Here's how the part is built. I have some questions about the finished solid (model axes, mm). Face numbers are marked on the shaded views. A direction names the side the tool comes from. Coordinates: 2 decimals unless noted, no trailing zeros. Write each loop counter-clockwise with the first axis right and the second up, starting at its lowest first coordinate (ties: lowest second). Pieces come first, ordered by that corner, then holes.
(1) Imagine slicing it at C-C, the plane x = -12.5. List the corners of the cut face in (y, z) for me, plus the area to 3 significant figures.
(2) Imagine slicing it at D-D, the plane z = -7.25. List the corners of the cut face in (x, y) for me.
(3) Imagine slicing it at B-B, the plane x = -7.5. List the corners of the cut face in (y, z) for me, plus the area to 3 significant figures.
(4) Imagine slicing it at A-A, the plane y = 51. List the corners of the cut face in (x, z) for me.
(5) Which directions (+Z, -Z, +X, -X, +Y, -Y) give clear straight access to the entire face, cutting with the end or side of a thin tool? Please do the marked faces 4, 5 and 6.
(6) For pin 1 Ø1 at (y, z) = (38.5, 6) entering from -X; pin 2 Ø1.6 at (x, z) = (24.5, -0.5) entering from +Y; pin 3 Ø4.5 at (y, z) = (30.5, 8.5) entering from +X, each with a flat end and sliding along its axis, tell me the tip position at first contact or that it passes through.
(7) Please list where these lines run through material, in increasing order: probe 1 along Y at (x, z) = (-13.25, -5); probe 2 along X at (y, z) = (2.75, 0); probe 3 along Z at (x, y) = (-10.75, 4).
(8) Thinking about a two-plate mould opening in Y: for the marked faces 1, 2 and 3, which applies, released by +Y, released by -Y, zero draft, split by the parting line, or undercut?
```python
from build123d import *

# Parameters (mm, degrees)
ESQUISSE1_W                                 = 45
ESQUISSE1_H                                 = 30
BOSS_EXTRU_1_DEPTH                          = 8
ESQUISSE5_W                                 = 30
ESQUISSE5_H                                 = 48
BOSS_EXTRU_3_DEPTH                          = 32
ENL_V_MAT_EXTRU_1_DEPTH                     = 27
ESQUISSE14_W                                = 6
ESQUISSE14_H                                = 8
ENL_V_MAT_EXTRU_2_DEPTH                     = 65.600696591
D_GAGEMENT_M31_D                            = 3.2
D_GAGEMENT_M31_DEPTH                        = 7
D_GAGEMENT_M31_TIP                          = 0.96137699
ESQUISSE16_W                                = 30
ESQUISSE16_H                                = 48
ESQUISSE16_R                                = 3.5
BOSS_EXTRU_4_DEPTH                          = 5
CONG_1_R                                    = 2
ESQUISSE17_W                                = 10
ESQUISSE17_H                                = 10
ENL_V_MAT_EXTRU_3_DEPTH                     = 2
BOSS_EXTRU_5_START                          = 2
ESQUISSE18_R                                = 6
ESQUISSE18_R_2                              = 3.5
BOSS_EXTRU_5_DEPTH                          = 2
FRAISAGE_POUR_VIS_T_TE_FRAIS_E_M31_AT_COUNT = 2
FRAISAGE_POUR_VIS_T_TE_FRAIS_E_M31_AT_PITCH = 15
ESQUISSE24_W                                = 8
ESQUISSE24_H                                = 8
BOSS_EXTRU_6_DEPTH                          = 2.6


with BuildPart() as part:
    # Esquisse1 → Boss.-Extru.1 (new body)
    with BuildSketch(Plane(origin=(0, 0, 0), x_dir=(1, 0, 0), z_dir=(0, 1, 0))):
        with Locations((6, 0)):
            Rectangle(ESQUISSE1_W, ESQUISSE1_H)
    extrude(amount=BOSS_EXTRU_1_DEPTH)

    # Esquisse5 → Boss.-Extru.3 (add)
    with BuildSketch(Plane.ZY.offset(16.5)):
        with Locations((0, 32)):
            Rectangle(ESQUISSE5_W, ESQUISSE5_H)
    extrude(amount=-BOSS_EXTRU_3_DEPTH)

    # Esquisse6 → Enl_v. mat.-Extru.1 (cut)
    with BuildSketch(Plane.ZY.offset(16.5)):
        Polygon((10.25, 48), (4, 48), (4, 56), (-4, 56), (-4, 48), (-10.25, 48), (-10.25, 8), (10.25, 8), align=None)
    extrude(amount=-ENL_V_MAT_EXTRU_1_DEPTH, mode=Mode.SUBTRACT)

    # Esquisse14 → Enl_v. mat.-Extru.2 (cut, through all)
    with BuildSketch(Plane(origin=(0, 56, 0), x_dir=(1, 0, 0), z_dir=(0, 1, 0))):
        with Locations((16.5, 0)):
            Rectangle(ESQUISSE14_W, ESQUISSE14_H)
    extrude(amount=-ENL_V_MAT_EXTRU_2_DEPTH, mode=Mode.SUBTRACT)

    # D_gagement M31
    with Locations(Plane.ZY.offset(16.5)):
        with Locations((5, 4), (-5, 4)):
            Hole(D_GAGEMENT_M31_D / 2, depth=D_GAGEMENT_M31_DEPTH)
            with Locations((0, 0, -(D_GAGEMENT_M31_DEPTH + D_GAGEMENT_M31_TIP / 2))):  # 118° drill point
                Cone(0, D_GAGEMENT_M31_D / 2, D_GAGEMENT_M31_TIP, mode=Mode.SUBTRACT)

    # Esquisse16 → Boss.-Extru.4 (add)
    with BuildSketch(Plane(origin=(28.5, 0, 0), x_dir=(0, 0, -1), z_dir=(1, 0, 0))):
        with Locations((0, 32)):
            Rectangle(ESQUISSE16_W, ESQUISSE16_H)
        with Locations((0, 38)):
            Circle(ESQUISSE16_R, mode=Mode.SUBTRACT)
    extrude(amount=-BOSS_EXTRU_4_DEPTH)

    # Cong_1
    cong_1_edges = [part.edges().sort_by_distance(p)[0] for p in [
        (19.5, 8, 15),
        (15.5, 8, -9.5),
        (15.5, 32, -15),
        (15.5, 56, 9.5),
        (-0.5, 56, -15),
        (15.5, 32, 15),
        (-0.5, 56, 15),
        (-16.5, 56, 9.5),
        (-16.5, 56, -9.5),
        (15.5, 8, 9.5),
        (15.5, 56, -9.5),
        (28.5, 28, 15),
        (-16.5, 28, 15),
        (-16.5, 28, -15),
        (28.5, 28, -15),
        (19.5, 8, -15),
        (23.5, 32, 15),
        (23.5, 56, 0),
        (26, 56, 15),
        (23.5, 32, -15),
        (26, 56, -15),
        (23.5, 8, 0),
        (28.5, 56, 0),
    ]]
    fillet(cong_1_edges, radius=CONG_1_R)

    # Esquisse17 → Enl_v. mat.-Extru.3 (cut)
    with BuildSketch(Plane.ZY.offset(-23.5)):
        with Locations((0, 38)):
            Rectangle(ESQUISSE17_W, ESQUISSE17_H)
    extrude(amount=-ENL_V_MAT_EXTRU_3_DEPTH, mode=Mode.SUBTRACT)

    # Esquisse18 → Boss.-Extru.5 (add)
    with BuildSketch(Plane(origin=(28.5, 0, 0), x_dir=(0, 0, -1), z_dir=(1, 0, 0)).offset(BOSS_EXTRU_5_START)):
        with Locations(Location((0, 38, 0), (0, 0, 180))):
            Circle(ESQUISSE18_R)
        with Locations((0, 38)):
            Circle(ESQUISSE18_R_2, mode=Mode.SUBTRACT)
    extrude(amount=-BOSS_EXTRU_5_DEPTH)

    # Esquisse23 → Fraisage pour vis _ t_te frais_e M31 (revolve, cut)
    with BuildSketch(Plane(origin=(-7.5, 8, 0), x_dir=(0, 0, 1), z_dir=(1, 0, 0))):
        Polygon((0, 0), (0, 8), (1.7, 8), (1.7, 1.45), (3.15, 0), align=None)
    fraisage_pour_vis_t_te_frais_e_m31 = revolve(axis=Axis((-7.5, 14.35, 0), (0, -1, 0)), mode=Mode.SUBTRACT)

    # Fraisage pour vis _ t_te frais_e M31 at: Fraisage pour vis _ t_te frais_e M31 ×2
    with Locations(*[(i * FRAISAGE_POUR_VIS_T_TE_FRAIS_E_M31_AT_PITCH, 0, 0) for i in range(1, FRAISAGE_POUR_VIS_T_TE_FRAIS_E_M31_AT_COUNT)]):
        add(fraisage_pour_vis_t_te_frais_e_m31, mode=Mode.SUBTRACT)

    # Esquisse24 → Boss.-Extru.6 (add)
    with BuildSketch(Plane.ZY.offset(-10.5)):
        with Locations((0, 52)):
            Rectangle(ESQUISSE24_W, ESQUISSE24_H)
    extrude(amount=BOSS_EXTRU_6_DEPTH)


solid = part.part
```
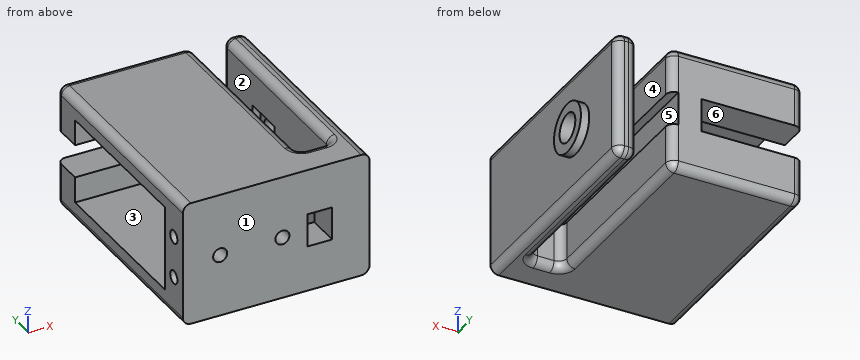
Recorded:
1. outline: (0, -15) - (54, -15) arc R2 ccw to (56, -13) - (56, -4) - (48, -4) - (48, -10.25) - (8, -10.25) - (8, 10.25) - (48, 10.25) - (48, 4) - (56, 4) - (56, 13) arc R2 ccw to (54, 15) - (0, 15) - close; hole circle Ø3.2 at (4, -5); hole circle Ø3.2 at (4, 5)
1. area: 778 mm2
2. outline: (-16.5, 0) - (28.5, 0) - (28.5, 54) arc R2 ccw to (26.5, 56) - (25.5, 56) arc R2 ccw to (23.5, 54) - (23.5, 10) arc R2 cw to (21.5, 8) - (17.5, 8) arc R2 cw to (15.5, 10) - (15.5, 54) arc R2 ccw to (13.5, 56) - (-14.5, 56) arc R2 ccw to (-16.5, 54) - (-16.5, 48) - (10.5, 48) - (10.5, 8) - (-16.5, 8) - close
3. outline: (0, -15) - (54, -15) arc R2 ccw to (56, -13) - (56, -4) - (48, -4) - (48, -10.25) - (8, -10.25) - (8, -3.15) - (6.55, -1.7) - (0, -1.7) - close; (0, 1.7) - (6.55, 1.7) - (8, 3.15) - (8, 10.25) - (48, 10.25) - (48, 4) - (56, 4) - (56, 13) arc R2 ccw to (54, 15) - (0, 15) - close
3. area: 765 mm2
4. outline: (-16.5, -13) arc R2 ccw to (-14.5, -15) - (13.5, -15) arc R2 ccw to (15.5, -13) - (15.5, -4) - (13.5, -4) - (13.5, 4) - (15.5, 4) - (15.5, 13) arc R2 ccw to (13.5, 15) - (-14.5, 15) arc R2 ccw to (-16.5, 13) - (-16.5, 4) - (7.9, 4) - (7.9, -4) - (-16.5, -4) - close; (23.5, -13) arc R2 ccw to (25.5, -15) - (26.5, -15) arc R2 ccw to (28.5, -13) - (28.5, 13) arc R2 ccw to (26.5, 15) - (25.5, 15) arc R2 ccw to (23.5, 13) - close
5. face 4: +Z, -Z, +Y
5. face 5: +Y, -Y
5. face 6: -X, +Y
6. pin 1: stops at x = 10.5
6. pin 2: stops at y = 55.99
6. pin 3: stops at x = 28.5
7. probe 1: y = 0 to 2.4, 5.6 to 8, 48 to 56
7. probe 2: x = -16.5 to -9.2, -5.8 to 5.8, 9.2 to 13.5, 19.5 to 28.5
7. probe 3: z = -15 to -6.6, -3.4 to 3.4, 6.6 to 15
8. face 1: released by -Y
8. face 2: zero draft
8. face 3: undercut
